Geometry check sheet. Reference: the model listing, model coordinates, mm. Face numbers are marked on the shaded views. A direction names the side the tool comes from. Round coordinates to 2 decimals unless told otherwise and drop trailing zeros. Loops run counter-clockwise (first coordinate to the right, second up) from the corner with the lowest first, then second, coordinate; pieces in that order, holes last.
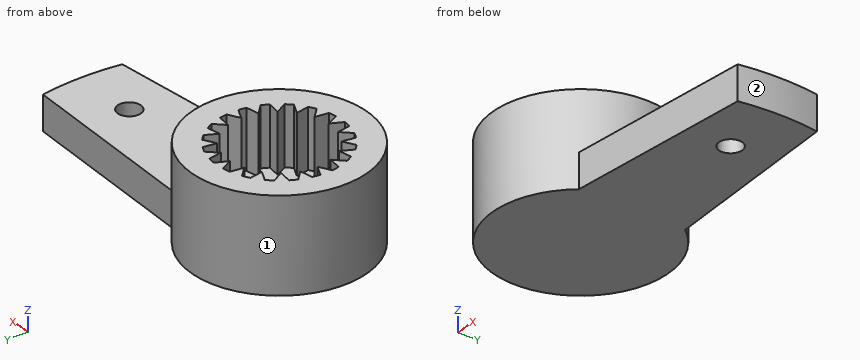
```python
from build123d import *

# Parameters (mm, degrees)
BOSS_EXTRUDE2_DEPTH = 1.4
SKETCH6_R           = 0.47083328
CUT_EXTRUDE1_DEPTH  = 12.066142252
SKETCH8_R           = 3.549999952
BOSS_EXTRUDE3_DEPTH = 3.8
CUT_EXTRUDE2_START  = -2.4
SKETCH9_R           = 2.549999919
CUT_EXTRUDE2_DEPTH  = 2.4
BOSS_EXTRUDE4_START = -2.4
BOSS_EXTRUDE4_DEPTH = 2.4


with BuildPart() as part:
    # Sketch5 → Boss-Extrude2 (new body)
    with BuildSketch(Plane.XY.offset(-2.4)):
        with BuildLine():
            Line((2.776387215, 2.212277889), (10.622617722, 1.649999976))
            ThreePointArc((10.622617722, 1.649999976), (10.75199195, 0), (10.622617722, -1.649999976))
            Line((10.622617722, -1.649999976), (2.776387215, -2.212277889))
            ThreePointArc((2.776387215, -2.212277889), (3.549999952, 0), (2.776387215, 2.212277889))
        make_face()
    extrude(amount=-BOSS_EXTRUDE2_DEPTH)

    # Sketch6 → Cut-Extrude1 (cut, through all)
    with BuildSketch(Plane.XY.offset(-2.4)):
        with Locations((8.100000381, 0)):
            Circle(SKETCH6_R)
    extrude(amount=-CUT_EXTRUDE1_DEPTH, mode=Mode.SUBTRACT)

    # Sketch8 → Boss-Extrude3 (add)
    with BuildSketch(Plane.XY):
        Circle(SKETCH8_R)
    extrude(amount=-BOSS_EXTRUDE3_DEPTH)

    # Sketch9 → Cut-Extrude2 (cut)
    with BuildSketch(Plane.XY.offset(CUT_EXTRUDE2_START)):
        Circle(SKETCH9_R)
    extrude(amount=CUT_EXTRUDE2_DEPTH, mode=Mode.SUBTRACT)

    # Sketch7 → Boss-Extrude4 (add)
    with BuildSketch(Plane.XY.offset(BOSS_EXTRUDE4_START)):
        with BuildLine():
            Line((-0.244697916, 2.538232164), (0, 2.049999952))
            Line((0, 2.049999952), (0.244697916, 2.538232164))
            ThreePointArc((0.244697916, 2.538232164), (0, 2.549999919), (-0.244697916, 2.538232164))
        make_face()
        with BuildLine():
            Line((0.551635326, 2.489618054), (0.633484824, 1.949665813))
            Line((0.633484824, 1.949665813), (1.017078422, 2.338386424))
            ThreePointArc((1.017078422, 2.338386424), (0.787993311, 2.42519404), (0.551635326, 2.489618054))
        make_face()
        with BuildLine():
            Line((1.29397066, 2.197302783), (1.204959739, 1.6584848))
            Line((1.204959739, 1.6584848), (1.689900206, 1.90964313))
            ThreePointArc((1.689900206, 1.90964313), (1.498852346, 2.06299327), (1.29397066, 2.197302783))
        make_face()
        with BuildLine():
            Line((1.90964313, 1.689900206), (1.6584848, 1.204959739))
            Line((1.6584848, 1.204959739), (2.197302783, 1.29397066))
            ThreePointArc((2.197302783, 1.29397066), (2.06299327, 1.498852346), (1.90964313, 1.689900206))
        make_face()
        with BuildLine():
            Line((2.338386424, 1.017078422), (1.949665813, 0.633484824))
            Line((1.949665813, 0.633484824), (2.489618054, 0.551635326))
            ThreePointArc((2.489618054, 0.551635326), (2.42519404, 0.787993311), (2.338386424, 1.017078422))
        make_face()
        with BuildLine():
            Line((2.538232164, 0.244697916), (2.049999952, 0))
            Line((2.049999952, 0), (2.538232164, -0.244697916))
            ThreePointArc((2.538232164, -0.244697916), (2.549999919, 0), (2.538232164, 0.244697916))
        make_face()
        with BuildLine():
            Line((2.489618054, -0.551635326), (1.949665813, -0.633484824))
            Line((1.949665813, -0.633484824), (2.338386424, -1.017078422))
            ThreePointArc((2.338386424, -1.017078422), (2.42519404, -0.787993311), (2.489618054, -0.551635326))
        make_face()
        with BuildLine():
            Line((2.197302783, -1.29397066), (1.6584848, -1.204959739))
            Line((1.6584848, -1.204959739), (1.90964313, -1.689900206))
            ThreePointArc((1.90964313, -1.689900206), (2.06299327, -1.498852346), (2.197302783, -1.29397066))
        make_face()
        with BuildLine():
            Line((1.689900206, -1.90964313), (1.204959739, -1.6584848))
            Line((1.204959739, -1.6584848), (1.29397066, -2.197302783))
            ThreePointArc((1.29397066, -2.197302783), (1.498852346, -2.06299327), (1.689900206, -1.90964313))
        make_face()
        with BuildLine():
            Line((1.017078422, -2.338386424), (0.633484824, -1.949665813))
            Line((0.633484824, -1.949665813), (0.551635326, -2.489618054))
            ThreePointArc((0.551635326, -2.489618054), (0.787993311, -2.42519404), (1.017078422, -2.338386424))
        make_face()
        with BuildLine():
            Line((0.244697916, -2.538232164), (0, -2.049999952))
            Line((0, -2.049999952), (-0.244697916, -2.538232164))
            ThreePointArc((-0.244697916, -2.538232164), (0, -2.549999919), (0.244697916, -2.538232164))
        make_face()
        with BuildLine():
            Line((-0.551635326, -2.489618054), (-0.633484824, -1.949665813))
            Line((-0.633484824, -1.949665813), (-1.017078422, -2.338386424))
            ThreePointArc((-1.017078422, -2.338386424), (-0.787993311, -2.42519404), (-0.551635326, -2.489618054))
        make_face()
        with BuildLine():
            Line((-1.29397066, -2.197302783), (-1.204959739, -1.6584848))
            Line((-1.204959739, -1.6584848), (-1.689900206, -1.90964313))
            ThreePointArc((-1.689900206, -1.90964313), (-1.498852346, -2.06299327), (-1.29397066, -2.197302783))
        make_face()
        with BuildLine():
            Line((-1.90964313, -1.689900206), (-1.6584848, -1.204959739))
            Line((-1.6584848, -1.204959739), (-2.197302783, -1.29397066))
            ThreePointArc((-2.197302783, -1.29397066), (-2.06299327, -1.498852346), (-1.90964313, -1.689900206))
        make_face()
        with BuildLine():
            Line((-2.338386424, -1.017078422), (-1.949665813, -0.633484824))
            Line((-1.949665813, -0.633484824), (-2.489618054, -0.551635326))
            ThreePointArc((-2.489618054, -0.551635326), (-2.42519404, -0.787993311), (-2.338386424, -1.017078422))
        make_face()
        with BuildLine():
            Line((-2.538232164, -0.244697916), (-2.049999952, 0))
            Line((-2.049999952, 0), (-2.538232164, 0.244697916))
            ThreePointArc((-2.538232164, 0.244697916), (-2.549999919, 0), (-2.538232164, -0.244697916))
        make_face()
        with BuildLine():
            Line((-2.489618054, 0.551635326), (-1.949665813, 0.633484824))
            Line((-1.949665813, 0.633484824), (-2.338386424, 1.017078422))
            ThreePointArc((-2.338386424, 1.017078422), (-2.42519404, 0.787993311), (-2.489618054, 0.551635326))
        make_face()
        with BuildLine():
            Line((-2.197302783, 1.29397066), (-1.6584848, 1.204959739))
            Line((-1.6584848, 1.204959739), (-1.90964313, 1.689900206))
            ThreePointArc((-1.90964313, 1.689900206), (-2.06299327, 1.498852346), (-2.197302783, 1.29397066))
        make_face()
        with BuildLine():
            Line((-1.689900206, 1.90964313), (-1.204959739, 1.6584848))
            Line((-1.204959739, 1.6584848), (-1.29397066, 2.197302783))
            ThreePointArc((-1.29397066, 2.197302783), (-1.498852346, 2.06299327), (-1.689900206, 1.90964313))
        make_face()
        with BuildLine():
            Line((-1.017078422, 2.338386424), (-0.633484824, 1.949665813))
            Line((-0.633484824, 1.949665813), (-0.551635326, 2.489618054))
            ThreePointArc((-0.551635326, 2.489618054), (-0.787993311, 2.42519404), (-1.017078422, 2.338386424))
        make_face()
    extrude(amount=BOSS_EXTRUDE4_DEPTH)


solid = part.part
```
1) Gauge pin test, flat ends, axial feed: pin 1 (1 mm diameter, centred on x = 6.5, y = -2.5, fed in from -Z); pin 2 (1.5 mm diameter, centred on x = 3.5, z = -2.5, fed in from +Y) (3 decimals); pin 3 (1 mm diameter, centred on y = 2.5, z = -1.5, fed in from -X); pin 4 (2 mm diameter, centred on x = 6, z = -2.5, fed in from +Y). Record the tip position at first contact, or that the pin passes through.
Report:
pin 1: passes through
pin 2: stops at y = 2.245
pin 3: stops at x = -2.93
pin 4: stops at y = 2.05
2) Scan lines: line 1 along Z through (x, y) = (7, -1.5); line 2 along Y through (x, z) = (8.1, -3.4); line 3 along Y through (x, z) = (0.5, -2.7). Record each from-to range of solid material in increasing order.
Report:
line 1: z = -3.8 to -2.4
line 2: y = -1.83 to -0.47, 0.47 to 1.83
line 3: y = -3.51 to 3.51
3) Sectioned sample at C-C, the plane x = 5. Record the cut outline in (y, z).
Report:
outline: (-2.05, -3.8) - (2.05, -3.8) - (2.05, -2.4) - (-2.05, -2.4) - close
4) Sectioned sample at B-B, the plane y = 1.5. Record the cut outline in (x, z), then the cut area to 3 significant figures.
Report:
outline: (-3.22, -3.8) - (10.65, -3.8) - (10.65, -2.4) - (3.22, -2.4) - (3.22, 0) - (1.81, 0) - (1.81, -2.4) - (-1.81, -2.4) - (-1.81, 0) - (-3.22, 0) - close
area: 26.2 mm2
5) Sectioned sample at A-A, the plane x = 8.1. Record the cut outline in (y, z), then the cut area to 3 significant figures.
Report:
outline: (-1.83, -3.8) - (-0.47, -3.8) - (-0.47, -2.4) - (-1.83, -2.4) - close; (0.47, -3.8) - (1.83, -3.8) - (1.83, -2.4) - (0.47, -2.4) - close
area: 3.81 mm2
6) Access from +Z, -Z, +X, -X, +Y, -Y to the whole of each face (thin tool, end or side, straight path). Record for the marked faces 1 and 2.
Report:
face 1: +Z
face 2: +Z, -Z, +X
